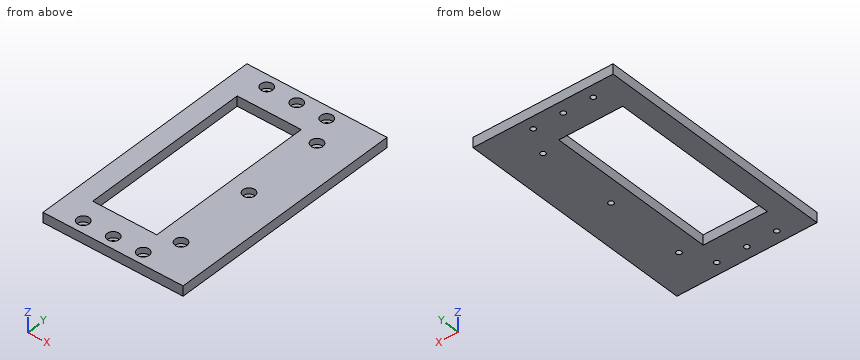
```python
from build123d import *

# Parameters (mm, degrees)
EXTRUDE_1_DEPTH           = 5
HOLE_WIZARD_2_D           = 2.6
HOLE_WIZARD_2_DEPTH       = 10
HOLE_WIZARD_2_CBORE_D     = 6
HOLE_WIZARD_2_CBORE_DEPTH = 3
SKETCH_8_W                = 32
SKETCH_8_H                = 85
CUT_EXTRUDE_1_DEPTH       = 73.284161474


with BuildPart() as part:
    # 草圖3 → 填料-伸長1 (new body)
    with BuildSketch(Plane.XY):
        Polygon((-30, 60), (-30, -60), (0, -60), (40, -60), (40, 60), (0, 60), align=None)
    extrude(amount=EXTRUDE_1_DEPTH)

    # 鑽孔2
    with Locations(Plane(origin=(-15, 54, 5), x_dir=(1, 0, 0), z_dir=(0, 0, 1))):
        with Locations((0, 0), (15, 0), (30, 0), (37, -14), (37, -94), (30, -108), (15, -108), (0, -108), (37, -54)):
            CounterBoreHole(HOLE_WIZARD_2_D / 2, HOLE_WIZARD_2_CBORE_D / 2, HOLE_WIZARD_2_CBORE_DEPTH, depth=HOLE_WIZARD_2_DEPTH)

    # 草圖8 → 除料-伸長1 (cut, through all)
    with BuildSketch(Plane.XY.offset(5)):
        with Locations((-4, 0)):
            Rectangle(SKETCH_8_W, SKETCH_8_H)
    extrude(amount=-CUT_EXTRUDE_1_DEPTH, mode=Mode.SUBTRACT)


solid = part.part
```
Geometry check sheet. Reference: the model listing, model coordinates, mm. Coordinates: 2 decimals unless noted, no trailing zeros. Write each loop counter-clockwise with the first axis right and the second up, starting at its lowest first coordinate (ties: lowest second). Pieces come first, ordered by that corner, then holes. Notation, with made-up numbers: M 22.5,70 L 73.5,70 A23 cw 73.5,80 Z; hole C 77,-5 d7. An arc over 180 degrees is marked long. Answer as a JSON object with one key per item and string values.
1. Scan lines: L1, parallel to Y at x = 15, z = 1.1; L2, parallel to Y at x = 22, z = 3.2; L3, parallel to Y at x = 22, z = 0.7. Record each from-to range of solid material in increasing order.
Answers below:
{"L1": "y = -60 to -55.3, -52.7 to 52.7, 55.3 to 60", "L2": "y = -60 to -43, -37 to -3, 3 to 37, 43 to 60", "L3": "y = -60 to -41.3, -38.7 to -1.3, 1.3 to 38.7, 41.3 to 60"}
2. Section check B-B, the plane y = 54. Enter the section's corners in (x, z), plus the area to 3 significant figures.
Answers below:
{"outline": "M -30,0 L -16.3,0 L -16.3,2 L -18,2 L -18,5 L -30,5 Z; M -13.7,0 L -1.3,0 L -1.3,2 L -3,2 L -3,5 L -12,5 L -12,2 L -13.7,2 Z; M 1.3,0 L 13.7,0 L 13.7,2 L 12,2 L 12,5 L 3,5 L 3,2 L 1.3,2 Z; M 16.3,0 L 40,0 L 40,5 L 18,5 L 18,2 L 16.3,2 Z", "area": "280 mm²"}
3. Section check D-D, the plane z = 3.05. Give the number of separate pieces and of enclosed holes in the cut face, plus the area to 3 significant figures.
Answers below:
{"separate pieces": "1", "enclosed holes": "10", "area": "5,430 mm²"}
4. Go/stop test with flat-tipped pins: pin 1 Ø3 at (x, y) = (15, 54) entering from -Z; pin 2 Ø1.8 at (x, y) = (0.5, 52.5) entering from +Z. Record where each tip stops, or that it passes through.
Answers below:
{"pin 1": "stops at z = 0", "pin 2": "stops at z = 2"}
5. Section check C-C, the plane x = -9.5. Enter the section's corners in (y, z).
Answers below:
{"outline": "M -60,0 L -42.5,0 L -42.5,5 L -60,5 Z; M 42.5,0 L 60,0 L 60,5 L 42.5,5 Z"}
6. Section check A-A, the plane x = 0. Enter the section's corners in (y, z), plus the area to 3 significant figures.
Answers below:
{"outline": "M -60,0 L -55.3,0 L -55.3,2 L -57,2 L -57,5 L -60,5 Z; M -52.7,0 L -42.5,0 L -42.5,5 L -51,5 L -51,2 L -52.7,2 Z; M 42.5,0 L 52.7,0 L 52.7,2 L 51,2 L 51,5 L 42.5,5 Z; M 55.3,0 L 60,0 L 60,5 L 57,5 L 57,2 L 55.3,2 Z", "area": "129 mm²"}
